Can you work these out from the model? Positions are in its coordinate system, mm. A direction names the side the tool comes from. Coordinates: 2 decimals unless noted, no trailing zeros. Loops run counter-clockwise (first coordinate to the right, second up) from the corner with the lowest first, then second, coordinate; pieces in that order, holes last.
```python
from build123d import *

# Parameters (mm, degrees)
SKETCH_R     = 1.6
SKETCH_W     = 27.5
SKETCH_H     = 47.8
PAD_DEPTH    = 6
POCKET_DEPTH = 2.5
FILLET_R     = 6


with BuildPart() as part:
    # Sketch (on Face1 of ShapeBinder) → Pad (new body)
    with BuildSketch(Plane.XY):
        Polygon((266.5, -110.55), (291.5, -110.55), (305, -148.45), (291.5, -186.35), (266.5, -186.35), (253, -148.45), align=None)
        with Locations((270, -116.55)):
            Circle(SKETCH_R, mode=Mode.SUBTRACT)
        with Locations((288, -116.55)):
            Circle(SKETCH_R, mode=Mode.SUBTRACT)
        with Locations((299, -148.45)):
            Circle(SKETCH_R, mode=Mode.SUBTRACT)
        with Locations((259, -148.45)):
            Circle(SKETCH_R, mode=Mode.SUBTRACT)
        with Locations((270, -180.35)):
            Circle(SKETCH_R, mode=Mode.SUBTRACT)
        with Locations((288, -180.35)):
            Circle(SKETCH_R, mode=Mode.SUBTRACT)
        with Locations((279, -148.45)):
            Rectangle(SKETCH_W, SKETCH_H, mode=Mode.SUBTRACT)
    extrude(amount=PAD_DEPTH)

    # Sketch001 (on Face17 of Pad) → Pocket (cut)
    with BuildSketch(Plane(origin=(0, 0, 0), x_dir=(1, 0, 0), z_dir=(0, 0, -1))):
        Polygon((261.8, 146.833419), (261.8, 150.066581), (259, 151.683162), (256.2, 150.066581), (256.2, 146.833419), (259, 145.216838), align=None)
        Polygon((301.8, 146.833419), (301.8, 150.066581), (299, 151.683162), (296.2, 150.066581), (296.2, 146.833419), (299, 145.216838), align=None)
    extrude(amount=-POCKET_DEPTH, mode=Mode.SUBTRACT)

    # Fillet
    fillet_edges = [part.edges().sort_by_distance(p)[0] for p in [
        (291.5, -110.55, 3),
        (266.5, -110.55, 3),
        (253, -148.45, 3),
        (266.5, -186.35, 3),
        (291.5, -186.35, 3),
        (305, -148.45, 3),
    ]]
    fillet(fillet_edges, radius=FILLET_R)


solid = part.part
```
Item 1: Suppose I cut it at D-D, the plane y = -170.5. Please give me the cut outline in (x, z), plus the area to 3 significant figures.
Results are:
outline: (260.85, 0) - (265.25, 0) - (265.25, 6) - (260.85, 6) - close; (292.75, 0) - (297.15, 0) - (297.15, 6) - (292.75, 6) - close
area: 52.7 mm2
Item 2: Suppose I cut it at C-C, the plane x = 291.5. Please give me the cut outline in (y, z).
Results are:
outline: (-184.6, 0) - (-172.35, 0) - (-172.35, 6) - (-184.6, 6) - close; (-124.55, 0) - (-112.3, 0) - (-112.3, 6) - (-124.55, 6) - close
Item 3: Suppose I cut it at B-B, the plane y = -116.55. Please give me the cut outline in (x, z).
Results are:
outline: (264.36, 0) - (268.4, 0) - (268.4, 6) - (264.36, 6) - close; (271.6, 0) - (286.4, 0) - (286.4, 6) - (271.6, 6) - close; (289.6, 0) - (293.64, 0) - (293.64, 6) - (289.6, 6) - close
Item 4: Suppose I cut it at A-A, the plane z = 3.9. Please give me the cut outline in (x, y), plus the area to 3 significant figures.
Results are:
outline: (253.72, -150.46) - (265.08, -182.36) arc R6 ccw to (270.73, -186.35) - (287.27, -186.35) arc R6 ccw to (292.92, -182.36) - (304.28, -150.46) arc R6 ccw to (304.28, -146.44) - (292.92, -114.54) arc R6 ccw to (287.27, -110.55) - (270.73, -110.55) arc R6 ccw to (265.08, -114.54) - (253.72, -146.44) arc R6 ccw to start; hole circle Ø3.2 at (259, -148.45); hole (265.25, -172.35) - (292.75, -172.35) - (292.75, -124.55) - (265.25, -124.55) - close; hole circle Ø3.2 at (270, -180.35); hole circle Ø3.2 at (270, -116.55); hole circle Ø3.2 at (288, -180.35); hole circle Ø3.2 at (288, -116.55); hole circle Ø3.2 at (299, -148.45)
area: 1,540 mm2
Item 5: On a 3-axis mill with a long thin cutter (end or side, diameter ignored), from which of +Z, -Z, +X, -X, +Y, -Y can I reach the whole of each face in a straight line? I mean faces 1 (the face through (304.63, -148.42, 3.04)), 2 (the face through (298, -147, 2.5)). Say none if no direction works.
Results are:
face 1: +Z, -Z, +X
face 2: -Z
Item 6: I need wall thicknesses on line 1 along X through (y, z) = (-148.45, 3.55); line 2 along X through (y, z) = (-116.55, 4.4); line 3 along Y through (x, z) = (282.5, 1.4). Which ranges of each line are inside material? Lowest first, please.
Results are:
line 1: x = 253.37 to 257.4, 260.6 to 265.25, 292.75 to 297.4, 300.6 to 304.63
line 2: x = 264.36 to 268.4, 271.6 to 286.4, 289.6 to 293.64
line 3: y = -186.35 to -172.35, -124.55 to -110.55
Item 7: I'm going to push flat-ended pins straight in: P1, Ø3, axis at x = 288, y = -116.55, coming from the +Z side; P2, Ø2, axis at x = 290.5, z = 4, coming from the +Y side; P3, Ø1.8, axis at y = -151.5, z = 1.5, coming from the +X side; P4, Ø1.7, axis at x = 259, y = -147, coming from the -Z side. Where does each tip first touch, or does it pass through?
Results are:
P1: passes through
P2: stops at y = -110.98
P3: stops at x = 304.23
P4: stops at z = 2.5
Item 8: We'd pull the mould along X, two halves only. Please class faces 3 (the face through (257.62, -150.886, 1.232)), 4 (the face through (290.684, -111.617, 3.042)), 5 (the face through (257.58, -146.036, 1.232)), 6 (the face through (262, -148, 0)): +X half, -X half, draft (parallel to the pull), parting line (faces both ways), or undercut.
Results are:
face 3: undercut
face 4: +X half
face 5: undercut
face 6: draft
